Geometry check sheet. Reference: the model listing, model coordinates, mm. A direction names the side the tool comes from. Give positions to 0.01 mm unless a question says otherwise; leave off trailing zeros. Write each loop counter-clockwise with the first axis right and the second up, starting at its lowest first coordinate (ties: lowest second). Pieces come first, ordered by that corner, then holes.
(1) Depth check by flat-ended pin: P1, Ø1, axis at y = -7.5, z = -5, coming from the +X side; P2, Ø3.5, axis at y = -7.75, z = 0, coming from the -X side; P3, Ø4, axis at x = -0.5, y = -3.5, coming from the -Z side. Enter the tip coordinate at first touch or a pass-through.
(2) Cross-section at D-D (z = -8). Record the boundary of the cut face in (x, y).
(3) Tool access check on faces 4 (the cylindrical face through (1.75, 9.25, 0.07)), 5 (the flat face through (0, -2, -5)), 6 (the cylindrical face through (4.4, -4.5, -2.4)). Record the directions out of +Z, -Z, +X, -X, +Y, -Y that give a thin tool (end or side, any length) a straight path to the whole face; none if there is none.
(4) Mould release check, pull along Y, two halves, no side actions. Record for faces 1 (the flat face through (3.55, -2, -5)), 2 (the cylindrical face through (1.75, 0.07, -9.25)), 3 (the cylindrical face through (-2.5, -4.5, 2.4)): +Y half, -Y half, draft (parallel to the pull), parting line (faces both ways), or undercut.
(5) Cross-section at A-A (z = 1). Record the boundary of the cut face in (x, y).
(6) Thickness scan on line 1 along X through (y, z) = (5.25, 7.25); line 2 along Z through (x, y) = (-1.5, -2.5); line 3 along Y through (x, z) = (-1.5, 0). Record the ranges inside material, lowest first.
(7) Cross-section at C-C (y = -0.75). Record the boundary of the cut face in (x, z).
(8) Cross-section at B-B (y = 3). Record the boundary of the cut face in (x, z), and give its area (3 significant figures).
```python
from build123d import *

# Parameters (mm, degrees)
SKETCH1_R           = 11.025
BOSS_EXTRUDE1_DEPTH = 3.55
SKETCH2_R           = 5.1
BOSS_EXTRUDE2_DEPTH = 1.78
SKETCH3_R           = 5.1
BOSS_EXTRUDE3_DEPTH = 5
SKETCH5_R           = 4
CUT_EXTRUDE1_DEPTH  = 11.33
SKETCH6_R           = 1.5
CUT_EXTRUDE2_DEPTH  = 6.33
CIRPATTERN1_COUNT   = 4


with BuildPart() as part:
    # Sketch1 → Boss-Extrude1 (new body)
    with BuildSketch(Plane(origin=(0, 0, 0), x_dir=(0, 0, -1), z_dir=(1, 0, 0))):
        Circle(SKETCH1_R)
    extrude(amount=BOSS_EXTRUDE1_DEPTH)

    # Sketch2 → Boss-Extrude2 (add)
    with BuildSketch(Plane(origin=(3.55, 0, 0), x_dir=(0, 0, -1), z_dir=(1, 0, 0))):
        Circle(SKETCH2_R)
    extrude(amount=BOSS_EXTRUDE2_DEPTH)

    # Sketch3 → Boss-Extrude3 (add)
    with BuildSketch(Plane.ZY):
        Circle(SKETCH3_R)
    extrude(amount=BOSS_EXTRUDE3_DEPTH)

    # Sketch5 → Cut-Extrude1 (cut, through all)
    with BuildSketch(Plane.ZY.offset(5)):
        Circle(SKETCH5_R)
    extrude(amount=-CUT_EXTRUDE1_DEPTH, mode=Mode.SUBTRACT)

    # Sketch6 → Cut-Extrude2 (cut, through all)
    with BuildSketch(Plane.ZY):
        with Locations((-7.75, 0)):
            Circle(SKETCH6_R)
    cut_extrude2 = extrude(amount=-CUT_EXTRUDE2_DEPTH, mode=Mode.SUBTRACT)

    # CirPattern1: Cut-Extrude2 ×4 about axis
    cirpattern1_axis = Axis((0, 0, 0), (1, 0, 0))
    for i in range(1, CIRPATTERN1_COUNT):
        add(cut_extrude2.rotate(cirpattern1_axis, i * 360 / CIRPATTERN1_COUNT), mode=Mode.SUBTRACT)


solid = part.part
```
Reply:
1. P1: stops at x = 3.55
1. P2: stops at x = 0
1. P3: stops at z = -10.91
2. outline: (0, -7.59) - (3.55, -7.59) - (3.55, -1.48) - (0, -1.48) - close; (0, 1.48) - (3.55, 1.48) - (3.55, 7.59) - (0, 7.59) - close
3. face 4: +X, -X
3. face 5: -X
3. face 6: +X
4. face 1: draft
4. face 2: undercut
4. face 3: parting line
5. outline: (-5, -5) - (0, -5) - (0, -6.63) - (3.55, -6.63) - (3.55, -5) - (5.33, -5) - (5.33, -3.87) - (-5, -3.87) - close; (-5, 3.87) - (5.33, 3.87) - (5.33, 5) - (3.55, 5) - (3.55, 6.63) - (0, 6.63) - (0, 5) - (-5, 5) - close; (0, -10.98) - (3.55, -10.98) - (3.55, -8.87) - (0, -8.87) - close; (0, 8.87) - (3.55, 8.87) - (3.55, 10.98) - (0, 10.98) - close
6. line 1: x = 0 to 3.55
6. line 2: z = -4.45 to -3.12, 3.12 to 4.45
6. line 3: y = -5.1 to -4, 4 to 5.1
7. outline: (-5, -5.04) - (0, -5.04) - (0, -6.45) - (3.55, -6.45) - (3.55, -5.04) - (5.33, -5.04) - (5.33, -3.93) - (-5, -3.93) - close; (-5, 3.93) - (5.33, 3.93) - (5.33, 5.04) - (3.55, 5.04) - (3.55, 6.45) - (0, 6.45) - (0, 5.04) - (-5, 5.04) - close; (0, -11) - (3.55, -11) - (3.55, -9.05) - (0, -9.05) - close; (0, 9.05) - (3.55, 9.05) - (3.55, 11) - (0, 11) - close
8. outline: (-5, -4.12) - (0, -4.12) - (0, -10.61) - (3.55, -10.61) - (3.55, -4.12) - (5.33, -4.12) - (5.33, -2.65) - (-5, -2.65) - close; (-5, 2.65) - (5.33, 2.65) - (5.33, 4.12) - (3.55, 4.12) - (3.55, 10.61) - (0, 10.61) - (0, 4.12) - (-5, 4.12) - close
8. area: 76.6 mm2
